Could you check a few things on this model? Use its own coordinates, in mm. Face numbers are marked on the shaded views. A direction names the side the tool comes from. Round coordinates to 2 decimals unless told otherwise and drop trailing zeros. Loops run counter-clockwise (first coordinate to the right, second up) from the corner with the lowest first, then second, coordinate; pieces in that order, holes last. Notation, with made-up numbers: M 58.25,-21 L 62.25,-21 A37 cw 62.25,17 Z; hole C 9.25,86 d6. An arc over 180 degrees is marked long. Answer in a Markdown table with one row per item.
```python
from build123d import *

# Parameters (mm, degrees)
PAD_DEPTH         = 6.5
POCKET_DEPTH      = 1
SKETCH002_W       = 0.3
SKETCH002_H       = 1.2
SKETCH002_H_2     = 0.8
PAD001_DEPTH      = 1.58
PAD001_DEPTH_BACK = -0.8
SKETCH004_W       = 0.2
SKETCH004_H       = 0.75
PAD002_DEPTH      = 0.2
PAD003_DEPTH      = 2
PAD004_DEPTH      = 5.7


with BuildPart() as part:
    # Sketch → Pad (new body)
    with BuildSketch(Plane.XZ):
        with BuildLine():
            ThreePointArc((-2.89, 3.16), (-4.47, 1.58), (-2.89, 0))
            Line((-2.89, 0), (2.89, 0))
            ThreePointArc((2.89, 0), (4.47, 1.58), (2.89, 3.16))
            Line((2.89, 3.16), (-2.89, 3.16))
        make_face()
        with BuildLine():
            ThreePointArc((-2.89, 2.86), (-4.17, 1.58), (-2.89, 0.3))
            Line((-2.89, 0.3), (2.89, 0.3))
            ThreePointArc((2.89, 0.3), (4.17, 1.58), (2.89, 2.86))
            Line((2.89, 2.86), (-2.89, 2.86))
        make_face(mode=Mode.SUBTRACT)
    extrude(amount=PAD_DEPTH)

    # Sketch001 (on DatumPlane) → Pocket (cut)
    with BuildSketch(Plane(origin=(0, 0, 3.16), x_dir=(-1, 0, 0), z_dir=(0, 0, 1))):
        Polygon((-2.545, 0), (-2.545, 1.8), (-1.165, 1.8), (-1.165, 0.5), (1.165, 0.5), (1.165, 1.8), (2.545, 1.8), (2.545, 0), align=None)
    extrude(amount=-POCKET_DEPTH, mode=Mode.SUBTRACT)

    # Sketch002 (on DatumPlane) → Pad001 (join, two sides)
    with BuildSketch(Plane(origin=(0, 0, 0), x_dir=(1, 0, 0), z_dir=(0, 0, -1))) as pad001_sk:
        with Locations((-4.32, 5.2)):
            Rectangle(SKETCH002_W, SKETCH002_H)
        with Locations((4.32, 5.2)):
            Rectangle(SKETCH002_W, SKETCH002_H)
        with Locations((-4.32, 0.4)):
            Rectangle(SKETCH002_W, SKETCH002_H_2)
        with Locations((4.32, 0.4)):
            Rectangle(SKETCH002_W, SKETCH002_H_2)
    extrude(amount=-PAD001_DEPTH)
    extrude(pad001_sk.sketch, amount=-PAD001_DEPTH_BACK)

    # Sketch004 → Pad002 (join)
    with BuildSketch(Plane(origin=(0, 0, 0), x_dir=(1, 0, 0), z_dir=(0, 0, -1))):
        with Locations((-3.35, -0.035)):
            Rectangle(SKETCH004_W, SKETCH004_H)
        with Locations((-3.1, -0.035)):
            Rectangle(SKETCH004_W, SKETCH004_H)
        with Locations((-2.53, -0.035)):
            Rectangle(SKETCH004_W, SKETCH004_H)
        with Locations((-2.28, -0.035)):
            Rectangle(SKETCH004_W, SKETCH004_H)
        with Locations((-1.75, -0.035)):
            Rectangle(SKETCH004_W, SKETCH004_H)
        with Locations((-1.25, -0.035)):
            Rectangle(SKETCH004_W, SKETCH004_H)
        with Locations((-0.75, -0.035)):
            Rectangle(SKETCH004_W, SKETCH004_H)
        with Locations((-0.25, -0.035)):
            Rectangle(SKETCH004_W, SKETCH004_H)
        with Locations((3.35, -0.035)):
            Rectangle(SKETCH004_W, SKETCH004_H)
        with Locations((3.1, -0.035)):
            Rectangle(SKETCH004_W, SKETCH004_H)
        with Locations((2.53, -0.035)):
            Rectangle(SKETCH004_W, SKETCH004_H)
        with Locations((2.28, -0.035)):
            Rectangle(SKETCH004_W, SKETCH004_H)
        with Locations((1.75, -0.035)):
            Rectangle(SKETCH004_W, SKETCH004_H)
        with Locations((1.25, -0.035)):
            Rectangle(SKETCH004_W, SKETCH004_H)
        with Locations((0.75, -0.035)):
            Rectangle(SKETCH004_W, SKETCH004_H)
        with Locations((0.25, -0.035)):
            Rectangle(SKETCH004_W, SKETCH004_H)
    extrude(amount=-PAD002_DEPTH)

    # Sketch005 (on DatumPlane) → Pad003 (join)
    with BuildSketch(Plane(origin=(0, 0, 0), x_dir=(1, 0, 0), z_dir=(0, 1, 0))):
        with BuildLine():
            ThreePointArc((-2.95, -0.3), (-4.23, -1.58), (-2.95, -2.86))
            Line((-2.95, -2.86), (2.95, -2.86))
            ThreePointArc((2.95, -2.86), (4.23, -1.58), (2.95, -0.3))
            Line((2.95, -0.3), (-2.95, -0.3))
        make_face()
    extrude(amount=-PAD003_DEPTH)

    # Sketch006 (on DatumPlane) → Pad004 (join)
    with BuildSketch(Plane(origin=(0, 0, 0), x_dir=(1, 0, 0), z_dir=(0, 1, 0))):
        with BuildLine():
            ThreePointArc((-2.7, -1.28), (-3, -1.58), (-2.7, -1.88))
            Line((-2.7, -1.88), (2.7, -1.88))
            ThreePointArc((2.7, -1.88), (3, -1.58), (2.7, -1.28))
            Line((2.7, -1.28), (-2.7, -1.28))
        make_face()
    extrude(amount=-PAD004_DEPTH)


solid = part.part
```
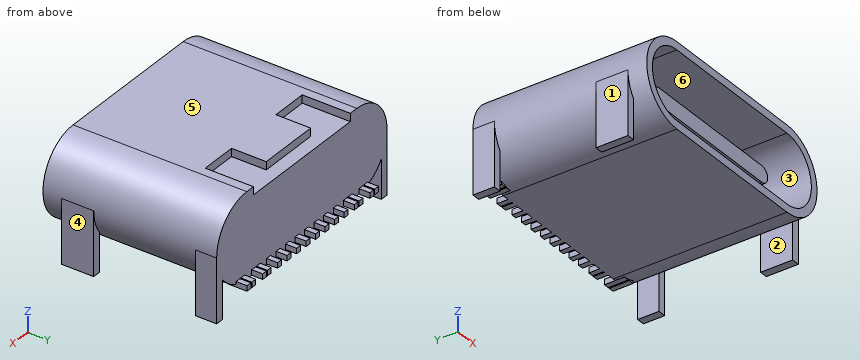
1) Will these pins go through, and if not, where does the flat tip stop? P1, Ø1.5, axis at x = -3, y = -1.5, coming from the -Z side; P2, Ø1, axis at x = -1, z = 2, coming from the -Y side; P3, Ø1.5, axis at x = -2.5, z = 2.5, coming from the +Y side.
Computed:
| item | result |
|---|---|
| P1 | stops at z = 0 |
| P2 | stops at y = -5.7 |
| P3 | stops at y = 0 |
2) I want a section at A-A, the plane y = -4.75. Please give me the cut outline in (x, z), plus the area to 3 significant figures.
Computed:
| item | result |
|---|---|
| outline | M -4.47,-0.8 L -4.17,-0.8 L -4.17,0.65 A1.58 ccw -2.89,0 L 2.89,0 A1.58 ccw 4.17,0.65 L 4.17,-0.8 L 4.47,-0.8 L 4.47,1.58 A1.58 ccw 2.89,3.16 L -2.89,3.16 A1.58 ccw -4.47,1.58 Z; M -2.7,1.28 L 2.7,1.28 A0.3 ccw 2.7,1.88 L -2.7,1.88 A0.3 ccw Z; hole M -2.89,0.3 L 2.89,0.3 A1.28 ccw 2.89,2.86 L -2.89,2.86 A1.28 ccw Z |
| area | 10.7 mm² |
3) I want a section at D-D, the plane z = 2.2. Please give me the cut outline in (x, y).
Computed:
| item | result |
|---|---|
| outline | M -4.34,-6.5 L -4.01,-6.5 L -4.01,-2 L 4.01,-2 L 4.01,-6.5 L 4.34,-6.5 L 4.34,0 L -4.34,0 Z |
4) I want a section at B-B, the plane y = -3.75. Please give me the cut outline in (x, z).
Computed:
| item | result |
|---|---|
| outline | M -2.89,0 L 2.89,0 A1.58 ccw 2.89,3.16 L -2.89,3.16 A1.58 ccw Z; M -2.7,1.28 L 2.7,1.28 A0.3 ccw 2.7,1.88 L -2.7,1.88 A0.3 ccw Z; hole M -2.89,0.3 L 2.89,0.3 A1.28 ccw 2.89,2.86 L -2.89,2.86 A1.28 ccw Z |
5) Which directions (+Z, -Z, +X, -X, +Y, -Y) give clear straight access to the entire face, cutting with the end or side of a thin tool? Please do the marked faces 1, 2 and 3.
Computed:
| item | result |
|---|---|
| face 1 | +Z, -Z, -X, +Y, -Y |
| face 2 | -Z, +Y, -Y |
| face 3 | -Y |
6) I need wall thicknesses on line 1 (Z direction, x = 0.25, y = -2.75); line 2 (X direction, y = -1.5, z = 3) (3 decimals); line 3 (Y direction, x = -2.5, z = 0.8). Which ranges of each line are inside material? Lowest first, please.
Computed:
| item | result |
|---|---|
| line 1 | z = 0 to 0.3, 1.28 to 1.88, 2.86 to 3.16 |
| line 2 | x = -3.583 to -2.545, -1.165 to 1.165, 2.545 to 3.583 |
| line 3 | y = -2 to 0 |
7) I want a section at C-C, the plane x = 1.75. Please give me the cut outline in (y, z).
Computed:
| item | result |
|---|---|
| outline | M -6.5,0 L 0.41,0 L 0.41,0.2 L 0,0.2 L 0,2.86 L -1.8,2.86 L -1.8,3.16 L -6.5,3.16 L -6.5,2.86 L -2,2.86 L -2,1.88 L -5.7,1.88 L -5.7,1.28 L -2,1.28 L -2,0.3 L -6.5,0.3 Z |
8) If we mould it in two halves opening along X, with no side actions, what happens to the marked faces 4, 5 and 6? For each: released by +X, released by -X, zero draft, split by the parting line, or undercut.
Computed:
| item | result |
|---|---|
| face 4 | released by +X |
| face 5 | zero draft |
| face 6 | undercut |
